Check sheet for the drawn part. Datum: minimum x, y, z corner. Units: mm. Give positions to 0.01 mm unless a question says otherwise; leave off trailing zeros. Loops run counter-clockwise (first coordinate to the right, second up) from the corner with the lowest first, then second, coordinate; pieces in that order, holes last. Notation, with made-up numbers: (75, 47.25) - (105, 47.25) arc R27 ccw to (105, 76.25) - close; hole circle Ø11 at (14, -17). An arc over 180 degrees is marked (long way). Use one line per item in the form item = value.
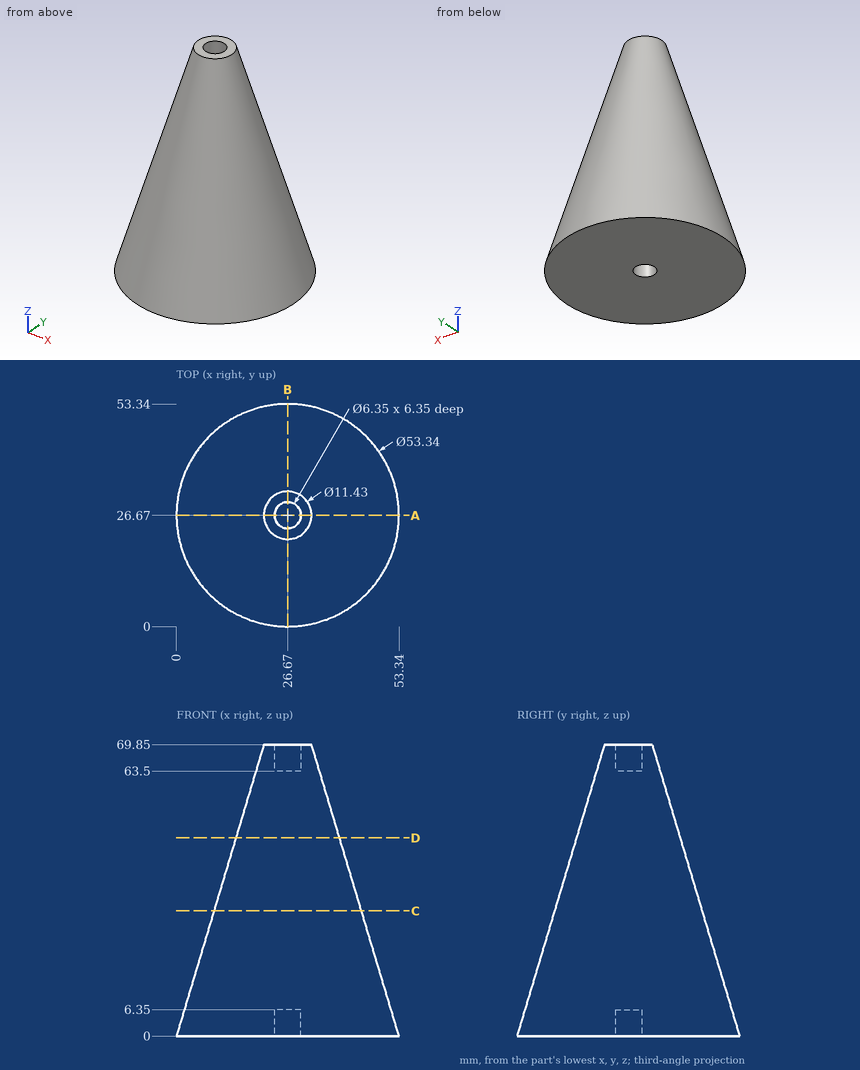
1. Depth check by flat-ended pin: pin 1 Ø7 at (x, y) = (27.5, 25) entering from +Z; pin 2 Ø1 at (x, z) = (23, 28.5) entering from -Y; pin 3 Ø8 at (x, z) = (18, 49) entering from -Y; pin 4 Ø5 at (x, y) = (26.67, 26.67) entering from +Z. Enter the tip coordinate at first touch or a pass-through.
Result set:
pin_1 = 69.85
pin_2 = 8.74
pin_3 = 15.22
pin_4 = 63.5
2. Scan lines: probe 1 along Y at (x, z) = (26.67, 67.25) (3 decimals); probe 2 along Y at (x, z) = (26.67, 66.25) (3 decimals); probe 3 along X at (y, z) = (26, 4). Record each from-to range of solid material in increasing order.
Result set:
probe_1 = 20.175 to 23.495, 29.845 to 33.165
probe_2 = 19.875 to 23.495, 29.845 to 33.465
probe_3 = 1.21 to 23.57, 29.77 to 52.13
3. Section check A-A, the plane y = 26.67. Record the cut outline in (x, z) (3 decimals), then the cut area to 3 significant figures.
Result set:
outline = (0, 0) - (23.495, 0) - (23.495, 6.35) - (29.845, 6.35) - (29.845, 0) - (53.34, 0) - (32.385, 69.85) - (29.845, 69.85) - (29.845, 63.5) - (23.495, 63.5) - (23.495, 69.85) - (20.955, 69.85) - close
area = 2,180 mm²
4. Section check D-D, the plane z = 47.5. Record the cut outline in (x, y).
Result set:
outline = circle Ø24.84 at (26.67, 26.67)
5. Section check C-C, the plane z = 30. Record the cut outline in (x, y), then the cut area to 3 significant figures.
Result set:
outline = circle Ø35.34 at (26.67, 26.67)
area = 981 mm²
